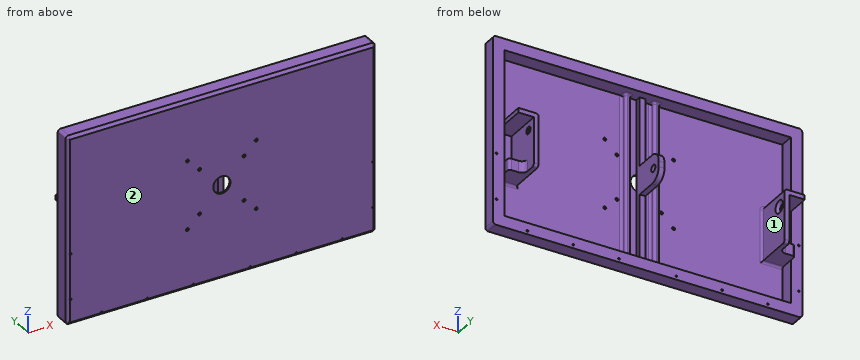
```python
from build123d import *

# Parameters (mm, degrees)
SKETCH1_W           = 540
SKETCH1_H           = 330
BOSS_EXTRUDE1_DEPTH = 3
SKETCH2_W           = 540
SKETCH2_H           = 330
SKETCH2_W_2         = 500
SKETCH2_H_2         = 290
BOSS_EXTRUDE2_DEPTH = 25
FILLET1_R           = 5
SKETCH4_R           = 1.6
CUT_EXTRUDE1_DEPTH  = 28
SKETCH5_R           = 15
CUT_EXTRUDE2_DEPTH  = 3
SKETCH6_W           = 10
SKETCH6_H           = 290
BOSS_EXTRUDE3_DEPTH = 10
FILLET3_R           = 4
CHAMFER1_SIZE       = 5
SKETCH7_R           = 2.6
CUT_EXTRUDE3_DEPTH  = 3
SKETCH9_R           = 2.6
CUT_EXTRUDE4_DEPTH  = 47
SKETCH11_W          = 8
SKETCH11_H          = 140
BOSS_EXTRUDE4_DEPTH = 66
SKETCH12_R          = 6.1
CUT_EXTRUDE5_DEPTH  = 8
SKETCH13_W          = 8
SKETCH13_H          = 69
SKETCH13_W_2        = 20
SKETCH13_H_2        = 40.75
BOSS_EXTRUDE5_DEPTH = 27
SKETCH15_W          = 8
SKETCH15_H          = 47
CUT_EXTRUDE6_DEPTH  = 66
FILLET4_R           = 4
FILLET5_R           = 10
FILLET6_R           = 5
FILLET7_R           = 5
CHAMFER2_SIZE       = 5
SKETCH19_W          = 10
SKETCH19_H          = 290
BOSS_EXTRUDE6_DEPTH = 10
SKETCH20_W          = 10
SKETCH20_H          = 50
BOSS_EXTRUDE7_DEPTH = 56
FILLET8_R           = 20
SKETCH21_R          = 6.1
CUT_EXTRUDE7_DEPTH  = 10


with BuildPart() as part:
    # Sketch1 → Boss-Extrude1 (new body)
    with BuildSketch(Plane(origin=(0, 0, 0), x_dir=(1, 0, 0), z_dir=(0, 1, 0))):
        Rectangle(SKETCH1_W, SKETCH1_H)
    extrude(amount=BOSS_EXTRUDE1_DEPTH)

    # Sketch2 → Boss-Extrude2 (add)
    with BuildSketch(Plane(origin=(0, 3, 0), x_dir=(1, 0, 0), z_dir=(0, 1, 0))):
        Rectangle(SKETCH2_W, SKETCH2_H)
        Rectangle(SKETCH2_W_2, SKETCH2_H_2, mode=Mode.SUBTRACT)
    extrude(amount=BOSS_EXTRUDE2_DEPTH)

    # Fillet1
    fillet1_edges = [part.edges().sort_by_distance(p)[0] for p in [
        (270, 14, 165),
        (-270, 14, 165),
        (-270, 14, -165),
        (270, 14, -165),
    ]]
    fillet(fillet1_edges, radius=FILLET1_R)

    # Sketch4 → Cut-Extrude1 (cut)
    with BuildSketch(Plane(origin=(0, 28, 0), x_dir=(1, 0, 0), z_dir=(0, 1, 0))):
        with Locations(Location((-264, 120, 0), (0, 0, 270))):
            Circle(SKETCH4_R)
        with Locations(Location((-264, 40, 0), (0, 0, 270))):
            Circle(SKETCH4_R)
        with Locations(Location((-210, 159, 0), (0, 0, 270))):
            Circle(SKETCH4_R)
        with Locations(Location((-130, 159, 0), (0, 0, 270))):
            Circle(SKETCH4_R)
        with Locations(Location((-50, 159, 0), (0, 0, 270))):
            Circle(SKETCH4_R)
        with Locations(Location((50, 159, 0), (0, 0, 90))):
            Circle(SKETCH4_R)
        with Locations(Location((130, 159, 0), (0, 0, 90))):
            Circle(SKETCH4_R)
        with Locations(Location((210, 159, 0), (0, 0, 90))):
            Circle(SKETCH4_R)
        with Locations(Location((264, 40, 0), (0, 0, 90))):
            Circle(SKETCH4_R)
        with Locations(Location((264, 120, 0), (0, 0, 90))):
            Circle(SKETCH4_R)
    extrude(amount=-CUT_EXTRUDE1_DEPTH, mode=Mode.SUBTRACT)

    # Sketch5 → Cut-Extrude2 (cut)
    with BuildSketch(Plane(origin=(0, 3, 0), x_dir=(1, 0, 0), z_dir=(0, 1, 0))):
        with Locations(Location((0, 0, 0), (0, 0, 270))):
            Circle(SKETCH5_R)
    extrude(amount=-CUT_EXTRUDE2_DEPTH, mode=Mode.SUBTRACT)

    # Sketch6 → Boss-Extrude3 (add)
    with BuildSketch(Plane(origin=(0, 3, 0), x_dir=(1, 0, 0), z_dir=(0, 1, 0))):
        with Locations((25, 0)):
            Rectangle(SKETCH6_W, SKETCH6_H)
        with Locations((-25, 0)):
            Rectangle(SKETCH6_W, SKETCH6_H)
    extrude(amount=BOSS_EXTRUDE3_DEPTH)

    # Fillet3
    fillet3_edges = [part.edges().sort_by_distance(p)[0] for p in [
        (30, 3, 0),
        (30, 8, 145),
        (30, 8, -145),
        (20, 3, 0),
        (20, 8, -145),
        (20, 8, 145),
        (30, 13, 0),
        (25, 13, -145),
        (20, 13, 0),
        (25, 13, 145),
        (-20, 3, 0),
        (-20, 8, 145),
        (-20, 8, -145),
        (-30, 3, 0),
        (-30, 8, -145),
        (-30, 8, 145),
        (-20, 13, 0),
        (-25, 13, -145),
        (-30, 13, 0),
        (-25, 13, 145),
    ]]
    fillet(fillet3_edges, radius=FILLET3_R)

    # Chamfer1
    # the kernel refuses this chamfer: 5 mm, written as the material it takes off along each edge
    with BuildSketch(Plane(origin=(-270, 0, -160), x_dir=(0, 1, 0), z_dir=(0, 0, 1)), Plane(origin=(270, 0, 160), x_dir=(0, 1, 0), z_dir=(0, 0, -1))) as chamfer1_piece_1:
        Polygon((CHAMFER1_SIZE, 0), (0, -CHAMFER1_SIZE), (0, 0), align=None)
    extrude(amount=320, mode=Mode.SUBTRACT)
    with BuildSketch(Plane(origin=(-265, 0, 165), x_dir=(0, 1, 0), z_dir=(1, 0, 0)), Plane(origin=(265, 0, -165), x_dir=(0, 1, 0), z_dir=(-1, 0, 0))) as chamfer1_piece_2:
        Polygon((CHAMFER1_SIZE, 0), (0, -CHAMFER1_SIZE), (0, 0), align=None)
    extrude(amount=530, mode=Mode.SUBTRACT)
    with BuildSketch(Plane(origin=(265, 0, -160), x_dir=(0, 0, -1), z_dir=(-1, 0, 0))) as chamfer1_piece_3:
        Polygon((5, -CHAMFER1_SIZE), (5 - CHAMFER1_SIZE, 0), (5, 0), align=None)
    revolve(axis=Axis((265, 0, -160), (0, -1, 0)), revolution_arc=90, mode=Mode.SUBTRACT)
    with BuildSketch(Plane(origin=(265, 0, 160), x_dir=(0, 0, 1), z_dir=(-1, 0, 0))) as chamfer1_piece_4:
        Polygon((5, CHAMFER1_SIZE), (5 - CHAMFER1_SIZE, 0), (5, 0), align=None)
    revolve(axis=Axis((265, 0, 160), (0, 1, 0)), revolution_arc=90, mode=Mode.SUBTRACT)
    with BuildSketch(Plane(origin=(-265, 0, 160), x_dir=(0, 0, 1), z_dir=(1, 0, 0))) as chamfer1_piece_5:
        Polygon((5, -CHAMFER1_SIZE), (5 - CHAMFER1_SIZE, 0), (5, 0), align=None)
    revolve(axis=Axis((-265, 0, 160), (0, -1, 0)), revolution_arc=90, mode=Mode.SUBTRACT)
    with BuildSketch(Plane(origin=(-265, 0, -160), x_dir=(0, 0, -1), z_dir=(1, 0, 0))) as chamfer1_piece_6:
        Polygon((5, CHAMFER1_SIZE), (5 - CHAMFER1_SIZE, 0), (5, 0), align=None)
    revolve(axis=Axis((-265, 0, -160), (0, 1, 0)), revolution_arc=90, mode=Mode.SUBTRACT)

    # Sketch7 → Cut-Extrude3 (cut)
    with BuildSketch(Plane.XZ):
        with Locations(Location((-60, 60, 0), (0, 0, 270))):
            Circle(SKETCH7_R)
        with Locations(Location((60, 60, 0), (0, 0, 270))):
            Circle(SKETCH7_R)
        with Locations(Location((60, -60, 0), (0, 0, 270))):
            Circle(SKETCH7_R)
        with Locations(Location((-60, -60, 0), (0, 0, 270))):
            Circle(SKETCH7_R)
    extrude(amount=-CUT_EXTRUDE3_DEPTH, mode=Mode.SUBTRACT)

    # Sketch9 → Cut-Extrude4 (cut)
    with BuildSketch(Plane.XZ):
        with Locations(Location((-38.890872965, 38.890872965, 0), (0, 0, 270))):
            Circle(SKETCH9_R)
        with Locations(Location((38.890872965, 38.890872965, 0), (0, 0, 270))):
            Circle(SKETCH9_R)
        with Locations(Location((38.890872965, -38.890872965, 0), (0, 0, 270))):
            Circle(SKETCH9_R)
        with Locations(Location((-38.890872965, -38.890872965, 0), (0, 0, 270))):
            Circle(SKETCH9_R)
    extrude(amount=-CUT_EXTRUDE4_DEPTH, mode=Mode.SUBTRACT)

    # Sketch11 → Boss-Extrude4 (add)
    with BuildSketch(Plane(origin=(0, 3, 0), x_dir=(1, 0, 0), z_dir=(0, 1, 0))):
        with Locations((-219, 0)):
            Rectangle(SKETCH11_W, SKETCH11_H)
    extrude(amount=BOSS_EXTRUDE4_DEPTH)

    # Sketch12 → Cut-Extrude5 (cut)
    with BuildSketch(Plane.ZY.offset(223)):
        with Locations((0, 53)):
            Circle(SKETCH12_R)
    extrude(amount=-CUT_EXTRUDE5_DEPTH, mode=Mode.SUBTRACT)

    # Sketch13 → Boss-Extrude5 (add)
    with BuildSketch(Plane.ZY.offset(223)):
        with Locations((19, 34.5)):
            Rectangle(SKETCH13_W, SKETCH13_H)
        with Locations((-60, 20.375)):
            Rectangle(SKETCH13_W_2, SKETCH13_H_2)
    extrude(amount=BOSS_EXTRUDE5_DEPTH)

    # Sketch15 → Cut-Extrude6 (cut)
    with BuildSketch(Plane(origin=(0, 69, 0), x_dir=(1, 0, 0), z_dir=(0, 1, 0))):
        with Locations((-219, -46.5)):
            Rectangle(SKETCH15_W, SKETCH15_H)
    extrude(amount=-CUT_EXTRUDE6_DEPTH, mode=Mode.SUBTRACT)

    # Fillet4
    fillet4_edges = [part.edges().sort_by_distance(p)[0] for p in [
        (-232.5, 3, -70),
        (-232.5, 3, 23),
        (-215, 3, -23.5),
        (-215, 36, 23),
    ]]
    fillet(fillet4_edges, radius=FILLET4_R)

    # Fillet5
    fillet5_edges = [part.edges().sort_by_distance(p)[0] for p in [
        (-223, 40.75, -60),
    ]]
    fillet(fillet5_edges, radius=FILLET5_R)

    # Fillet6
    fillet6_edges = [part.edges().sort_by_distance(p)[0] for p in [
        (-250, 40.75, -60),
    ]]
    fillet(fillet6_edges, radius=FILLET6_R)

    # Fillet7
    fillet7_edges = [part.edges().sort_by_distance(p)[0] for p in [
        (-219, 69, -70),
    ]]
    fillet(fillet7_edges, radius=FILLET7_R)

    # Chamfer2
    chamfer2_edges = [part.edges().sort_by_distance(p)[0] for p in [
        (-215, 53, -6.1),
    ]]
    chamfer(chamfer2_edges, length=CHAMFER2_SIZE)

    # Mirror9: part across plane


with BuildPart() as part_1:
    add(part.part)
    add(part.part.mirror(Plane(origin=(0, 0, 0), x_dir=(0, 0, 1), z_dir=(1, 0, 0))))

    # Sketch19 → Boss-Extrude6 (add)
    with BuildSketch(Plane(origin=(0, 3, 0), x_dir=(1, 0, 0), z_dir=(0, 1, 0))):
        Rectangle(SKETCH19_W, SKETCH19_H)
    extrude(amount=BOSS_EXTRUDE6_DEPTH)

    # Sketch20 → Boss-Extrude7 (add)
    with BuildSketch(Plane(origin=(0, 13, 0), x_dir=(1, 0, 0), z_dir=(0, 1, 0))):
        Rectangle(SKETCH20_W, SKETCH20_H)
    extrude(amount=BOSS_EXTRUDE7_DEPTH)

    # Fillet8
    fillet8_edges = [part_1.edges().sort_by_distance(p)[0] for p in [
        (0, 69, 25),
        (0, 69, -25),
    ]]
    fillet(fillet8_edges, radius=FILLET8_R)

    # Sketch21 → Cut-Extrude7 (cut)
    with BuildSketch(Plane.ZY.offset(5)):
        with Locations((0, 53)):
            Circle(SKETCH21_R)
    extrude(amount=-CUT_EXTRUDE7_DEPTH, mode=Mode.SUBTRACT)


solid = part_1.part
```
Work out the finished part from the listing and answer in its coordinate system (mm). Face numbers are marked on the shaded views. Round coordinates to 2 decimals unless told otherwise and drop trailing zeros. Write each loop counter-clockwise with the first axis right and the second up, starting at its lowest first coordinate (ties: lowest second). Pieces come first, ordered by that corner, then holes.
1) Determine the mould class of the marked faces 1 and 2 for opening direction X: pulls with the +X half, pulls with the -X half, needs draft (parallel to the pull), parting line crosses it, or undercut.
2) Consider probe 1 along X at (y, z) = (36, -20); probe 2 along Z at (x, y) = (-264, 15.75); probe 3 along X at (y, z) = (17.5, -120). Determine where each line is inside the solid, lowest interval first.
3) Flat-ended cylindrical pins translate along their axes: P1, Ø20, axis at y = 51, z = -23, coming from the +X side; P2, Ø2.5, axis at y = 31.5, z = -57.5, coming from the -X side; P3, Ø2.5, axis at x = 130, z = -159, coming from the +Y side; P4, Ø3, axis at x = -126, z = -123, coming from the +Y side. Find the tip coordinate at first contact, or state that the pin passes through.
4) A cutting plane is placed at A-A on x = -147. Determine the outline of the cut face in (y, z), and give its area (4 significant figures).
Entries:
1. face 1: undercut
1. face 2: needs draft
2. probe 1: x = -223 to -215, -5 to 5, 215 to 223
2. probe 2: z = -165 to -121.6, -118.4 to -41.6, -38.4 to 165
2. probe 3: x = -270 to -265.6, -262.4 to -250, 250 to 262.4, 265.6 to 270
3. P1: stops at x = 223
3. P2: stops at x = -250
3. P3: passes through
3. P4: stops at y = 3
4. outline: (0, -160) - (5, -165) - (28, -165) - (28, -145) - (3, -145) - (3, 145) - (28, 145) - (28, 165) - (5, 165) - (0, 160) - close
4. area: 1,965 mm2
